Part model, mm, in its own coordinate system. Face numbers are marked on the shaded views. A direction names the side the tool comes from. Round coordinates to 2 decimals unless told otherwise and drop trailing zeros. Loops run counter-clockwise (first coordinate to the right, second up) from the corner with the lowest first, then second, coordinate; pieces in that order, holes last. Notation, with made-up numbers: (5.5, 81.5) -> (41.5, 81.5) arc R20 cw to (41.5, 119.5) -> close; hole circle Ø8 at (23, 9). An arc over 180 degrees is marked (long way). Answer as a JSON object with one key per item and string values. Group by question number.
from build123d import *

# Parameters (mm, degrees)
F0_R     = 1.6
F1_DEPTH = 2
F3_W     = 35.5
F3_H     = 18
F4_DEPTH = 17
F6_W     = 8
F6_H     = 3
F7_DEPTH = 2


with BuildPart() as f1:
    # F0 (on Top) → F1 (new body)
    with BuildSketch(Plane.XY):
        with BuildLine():
            Line((-29.21, -20.32), (29.21, -20.32))
            Line((29.21, -20.32), (29.21, 20.32))
            Line((29.21, 20.32), (0.5, 20.32))
            ThreePointArc((0.5, 20.32), (0, 19.82), (-0.5, 20.32))
            Line((-0.5, 20.32), (-29.21, 20.32))
            Line((-29.21, 20.32), (-29.21, -20.32))
        make_face()
        with Locations((-26.67, -17.78)):
            Circle(F0_R, mode=Mode.SUBTRACT)
        with Locations((26.67, -17.78)):
            Circle(F0_R, mode=Mode.SUBTRACT)
        with Locations((-26.67, 17.78)):
            Circle(F0_R, mode=Mode.SUBTRACT)
        with Locations((26.67, 17.78)):
            Circle(F0_R, mode=Mode.SUBTRACT)
        with BuildLine():
            ThreePointArc((-0.5, 20.32), (0, 19.82), (0.5, 20.32))
            Line((0.5, 20.32), (-0.5, 20.32))
        make_face()
        with BuildLine():
            Line((-0.5, 20.32), (0.5, 20.32))
            ThreePointArc((0.5, 20.32), (0, 20.82), (-0.5, 20.32))
        make_face()
    extrude(amount=F1_DEPTH)

    # F3 (on offset) → F4 (join)
    with BuildSketch(Plane.XY.offset(2)):
        with Locations((-11.46, -3.81)):
            Rectangle(F3_W, F3_H)
    extrude(amount=F4_DEPTH)

    # F6 (on offset) → F7 (join)
    with BuildSketch(Plane(origin=(-29.21, 0, 0), x_dir=(0, -1, 0), z_dir=(-1, 0, 0))):
        with Locations((3.81, 17.5)):
            Rectangle(F6_W, F6_H)
    extrude(amount=F7_DEPTH)


solid = f1.part
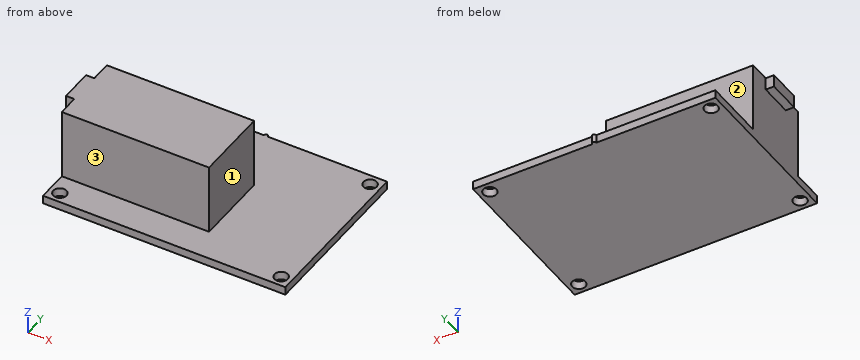
Item 1: Drop flat-ended pins along their axis: pin 1 Ø4 at (x, y) = (-26.67, -17.78) entering from +Z; pin 2 Ø3 at (y, z) = (4, 17) entering from +X; pin 3 Ø2 at (x, z) = (-16.5, 1.5) entering from +Y; pin 4 Ø6 at (y, z) = (11.5, 4) entering from +X. Give the stop position or say it passes through.
Item 2: Which spindle directions (+Z, -Z, +X, -X, +Y, -Y) get a long thin tool onto all of the face, cutting with end or side? Do the marked faces 1, 2 and 3. Say none if no direction does.
Item 3: Band-saw the part on C-C, the plane x = 5. List the corners of the cut face in (y, z), plus the area to 3 significant figures.
Item 4: Band-saw the part on B-B, the plane y = 17.78. List the corners of the cut face in (x, z), plus the area to 3 significant figures.
Item 5: Band-saw the part on D-D, the plane z = 13.75. List the corners of the cut face in (x, y), plus the area to 3 significant figures.
Item 6: Drill centre lines: line 1 (Y direction, x = 26.67, z = 0.45); line 2 (Z direction, x = 25, y = 14.5); line 3 (Y direction, x = -15, z = 1.5). Where is each one in solid material? Low to high.
Item 7: Band-saw the part on A-A, the plane x = -26.67. List the corners of the cut face in (y, z), plus the area to 3 significant figures.
Entries:
{
 "1": {"pin 1": "z = 2", "pin 2": "x = 6.29", "pin 3": "y = 20.32", "pin 4": "x = 29.21"},
 "2": {"face 1": "+Z, +X, +Y, -Y", "face 2": "+Z, +X, -X, +Y", "face 3": "+Z, +X, -X, -Y"},
 "3": {"outline": "(-20.32, 0) -> (20.32, 0) -> (20.32, 2) -> (5.19, 2) -> (5.19, 19) -> (-12.81, 19) -> (-12.81, 2) -> (-20.32, 2) -> close", "area": "387 mm²"},
 "4": {"outline": "(-29.21, 0) -> (-28.27, 0) -> (-28.27, 2) -> (-29.21, 2) -> close; (-25.07, 0) -> (25.07, 0) -> (25.07, 2) -> (-25.07, 2) -> close; (28.27, 0) -> (29.21, 0) -> (29.21, 2) -> (28.27, 2) -> close", "area": "104 mm²"},
 "5": {"outline": "(-29.21, -12.81) -> (6.29, -12.81) -> (6.29, 5.19) -> (-29.21, 5.19) -> close", "area": "639 mm²"},
 "6": {"line 1": "-20.32 to -19.38, -16.18 to 16.18, 19.38 to 20.32", "line 2": "0 to 2", "line 3": "-20.32 to 20.32"},
 "7": {"outline": "(-20.32, 0) -> (-19.38, 0) -> (-19.38, 2) -> (-20.32, 2) -> close; (-16.18, 0) -> (16.18, 0) -> (16.18, 2) -> (5.19, 2) -> (5.19, 19) -> (-12.81, 19) -> (-12.81, 2) -> (-16.18, 2) -> close; (19.38, 0) -> (20.32, 0) -> (20.32, 2) -> (19.38, 2) -> close", "area": "374 mm²"}
}
